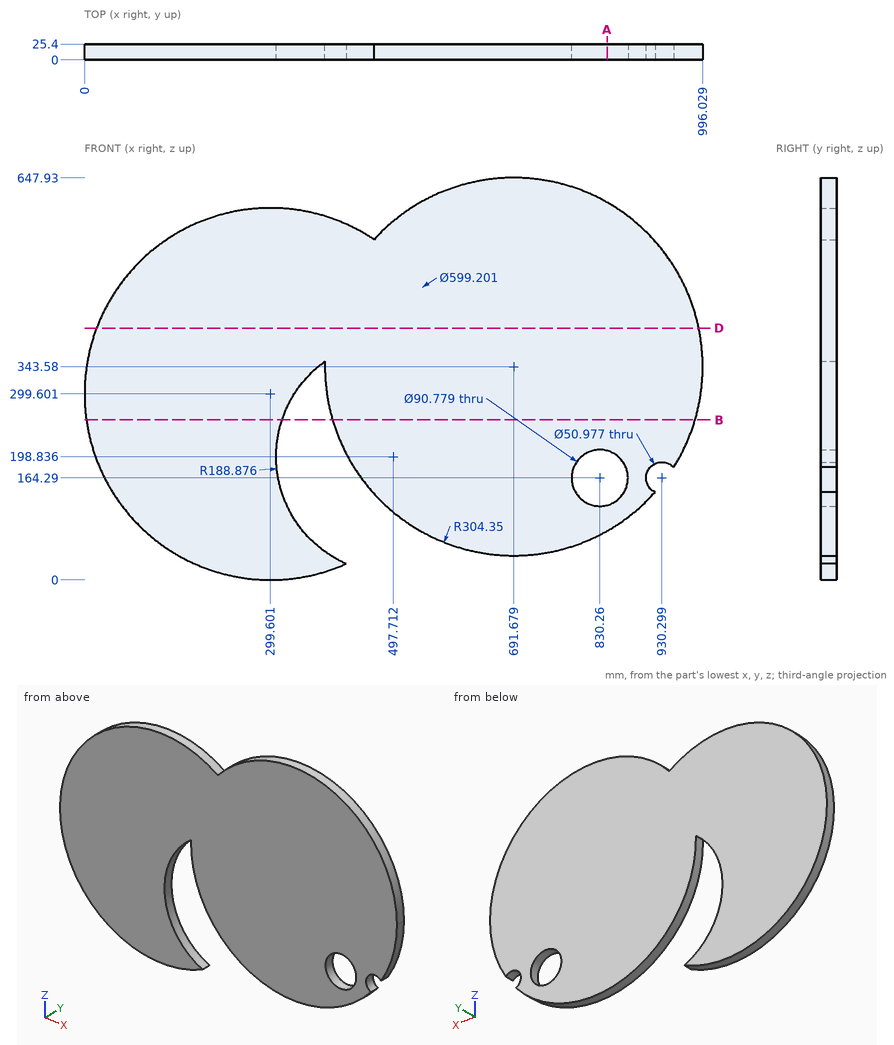
Input: dimensioned drawing with shaded views. Units: mm. Origin: part minimum x, y, z. Coordinates: 2 decimals unless noted, no trailing zeros. Write each loop counter-clockwise with the first axis right and the second up, starting at its lowest first coordinate (ties: lowest second). Pieces come first, ordered by that corner, then holes. Notation, with made-up numbers: (84.5, 77) -> (131.5, 77) arc R21 cw to (131.5, 103) -> close; hole circle Ø5 at (21.25, 19.25). An arc over 180 degrees is marked (long way). Return JSON: item names as keys, results as strings. Group by question number.
1) Section query A-A, the plane x = 842. Return loops of the section in (y, z) (1 decimal).
2) Ray query, line 1 along X through (y, z) = (2.25, 133) (1 decimal); line 2 along X through (y, z) = (11.5, 156.5) (1 decimal); line 3 along Z through (x, y) = (820.5, 18.75). Return the intervals inside material, ascending.
3) Section query D-D, the plane z = 405.5. Return loops of the section in (x, y), plus the area to 3 significant figures.
4) Section query B-B, the plane z = 258. Return loops of the section in (x, y).
5) Contact query for flat-ended pins moving along their axis: P1, Ø1, axis at x = 564.5, y = 2.5, coming from the -Z side; P2, Ø4, axis at x = 226.5, y = 21, coming from the +Z side; P3, Ø5, axis at x = 872, z = 237, coming from the -Y side; P4, Ø2, axis at y = 10.5, z = 410.5, coming from the +X side (1 decimal). Output: stop coordinate, or through.
From the geometry:
{
 "1": {"outline": "(0, 78.9) -> (25.4, 78.9) -> (25.4, 120.4) -> (0, 120.4) -> close; (0, 208.1) -> (25.4, 208.1) -> (25.4, 608.2) -> (0, 608.2) -> close"},
 "2": {"line 1": "50.6 to 320.7, 471.9 to 797.4, 863.1 to 911.4", "line 2": "36.4 to 313.6, 451.6 to 785.5, 875 to 906", "line 3": "67.84 to 119.96, 208.62 to 619.32"},
 "3": {"outline": "(19.34, 0) -> (989.66, 0) -> (989.66, 25.4) -> (19.34, 25.4) -> close", "area": "24,600 mm²"},
 "4": {"outline": "(2.9, 0) -> (318.34, 0) -> (318.34, 25.4) -> (2.9, 25.4) -> close; (399.61, 0) -> (983.75, 0) -> (983.75, 25.4) -> (399.61, 25.4) -> close"},
 "5": {"P1": "z = 66.85", "P2": "z = 590.64", "P3": "y = 0", "P4": "x = 988.8"}
}
